```python
from build123d import *

# Parameters (mm, degrees)
SKETCH1_R      = 3.175
EXTRUDE1_DEPTH = 18.25625
CHAMFER1_SIZE  = 0.635
EXTRUDE7_DEPTH = 26.793821935
FILLET1_R      = 0.79375
FILLET3_R      = 0.396875


with BuildPart() as part:
    # Sketch1 → Extrude1 (new, symmetric)
    with BuildSketch(Plane.XY):
        Circle(SKETCH1_R)
    extrude(amount=EXTRUDE1_DEPTH, both=True)

    # Chamfer1
    chamfer1_edges = [part.edges().sort_by_distance(p)[0] for p in [
        (-3.175, 0, -18.25625),
        (-3.175, 0, 18.25625),
    ]]
    chamfer(chamfer1_edges, length=CHAMFER1_SIZE)

    # Sketch13 → Extrude7 (cut, through all)
    with BuildSketch(Plane.XY.offset(-7.14375)):
        with BuildLine():
            Line((-1.5875, 2.749630657), (1.5875, 2.749630657))
            ThreePointArc((1.5875, 2.749630657), (0, 3.175), (-1.5875, 2.749630657))
        make_face()
    extrude(amount=EXTRUDE7_DEPTH, mode=Mode.SUBTRACT)

    # Fillet1
    # the kernel refuses this fillet: 0.79375 mm, written as the material it adds along each edge
    with BuildSketch(Plane(origin=(-3.571875, 2.749630657, -7.14375), x_dir=(0, 0, 1), z_dir=(1, 0, 0))) as fillet1_piece_1_section:
        with BuildLine():
            CenterArc((FILLET1_R, -FILLET1_R), FILLET1_R, 90, 90)
            Line((0, -FILLET1_R), (0, 0))
            Line((0, 0), (FILLET1_R, 0))
        make_face()
    fillet1_piece_1 = extrude(amount=7.14375, mode=Mode.PRIVATE)
    fillet1_piece_1 = fillet1_piece_1 & Plane(origin=(0, 0, -6.922980594), x_dir=(1, 0, 0), z_dir=(0, 0, 1)) * Cylinder(3.175, 18, mode=Mode.PRIVATE)
    add(fillet1_piece_1)

    # Fillet3
    fillet3_edges = [part.edges().sort_by_distance(p)[0] for p in [
        (1.5875, 2.749630657, 5.635625),
        (-1.5875, 2.749630657, 5.635625),
        (0, 3.175, -7.053089435),
        (-2.54, 0, -18.25625),
        (-3.175, 0, -17.62125),
        (-2.54, 0, 18.25625),
        (-1.5875, -2.749630657, 17.62125),
    ]]
    fillet(fillet3_edges, radius=FILLET3_R)


solid = part.part
```
The model under review builds one solid part; all positions refer to its coordinate system, in mm. A direction names the side the tool comes from. Give positions to 0.01 mm unless a question says otherwise; leave off trailing zeros. Write each loop counter-clockwise with the first axis right and the second up, starting at its lowest first coordinate (ties: lowest second). Pieces come first, ordered by that corner, then holes. Notation, with made-up numbers: (-13, -29) - (-6, -29) arc R22 cw to (-6, -3) - close; hole circle Ø6 at (-17.75, -37). An arc over 180 degrees is marked (long way). Answer in a Markdown table with one row per item. Add a question column.
1. Wall thickness on line 1 along Y through (x, z) = (2.75, -2.5); line 2 along Y through (x, z) = (-1.75, 2.5); line 3 along Z through (x, y) = (1, 2.25): over which ranges is each line inside the solid? List them lowest first. Write a range as [from, to].
2. Insertion check: P1, Ø3, axis at y = -1, z = -4, coming from the +X side (3 decimals); P2, Ø3.5, axis at x = 0.5, z = 9, coming from the +Y side. Each pin has a flat end and moves straight along its axis. Give the tip position at first contact, or say it passes through.
3. Tool access review of faces 1 (the flat face through (0, 2.75, 6)), 2 (the flat face through (0, 0, -18.256)): name each direction out of +Z, -Z, +X, -X, +Y, -Y from which nothing blocks a thin tool from reaching the whole face with its end or side.
4. We need section A-A on z = 0. Write out the cut boundary in (x, y) (3 decimals), then the cut area to 3 significant figures.
Ans:
| question | item | result |
|---|---|---|
| 1 | line 1 | y = [-1.59, 1.59] |
| 1 | line 2 | y = [-2.65, 2.65] |
| 1 | line 3 | z = [-18.25, 18.25] |
| 2 | P1 | stops at x = 3.175 |
| 2 | P2 | stops at y = 2.75 |
| 3 | face 1 | +Z, +X, -X, +Y |
| 3 | face 2 | -Z, +X, -X, +Y, -Y |
| 4 | outline | (-1.688, 2.689) arc R3.175 ccw (long way) to (1.688, 2.689) arc R0.397 ccw to (1.477, 2.75) - (-1.477, 2.75) arc R0.397 ccw to start |
| 4 | area | 30.8 mm^2 |
